Solid Edge part; units mm, degrees
sketch "Sketch1" plane through (0, 0, 0) normal (0, -1, 0) x (1, 0, 0)
  line L0 (2.75, 3) -> (2.75, 0)
  line L1 (2.75, 0) -> (1.8, 0)
  line L2 (1.8, 0) -> (1.5, -0.5196)
  line L3 (1.5, -0.5196) -> (1.5, -10)
  line L4 (1.5, -10) -> (0, -10)
  line L5 (1.25, 1.7) -> (0, 0.9783)
  line L6 (1.25, 3) -> (1.25, 1.7)
  line L7 (2.75, 3) -> (1.25, 3)
revolve "RevolvedProtrusion1" add sketch "Sketch1" angle 360 about axis through (0, 0, -6) along (0, 0, 1)
cosmetic_thread "Thread1"
chamfer "Chamfer_1" distance 0.25 angle 45 1 edges at (-1.5, 0, -10)
fillet "Round_1" radius 0.3 2 edges at (-2.75, 0, 0) (-2.75, 0, 3)
sketch "Sketch2" plane through (0, 0, 3) normal (0, 0, 1) x (0, 1, 0)
  line L0 (-1.25, 0.7217) -> (-1.25, -0.7217)
  line L1 (0, -1.4434) -> (-1.25, -0.7217)
  line L2 (1.25, -0.7217) -> (0, -1.4434)
  line L3 (1.25, 0.7217) -> (1.25, -0.7217)
  line L4 (0, 1.4434) -> (1.25, 0.7217)
  line L5 (-1.25, 0.7217) -> (0, 1.4434)
extrude "Cutout1" cut sketch "Sketch2" against normal up to vertex (1.3 mm away)
properties part number "STD-DIN912-M3x10" material "Galvanized steel"
Read the model definition and answer for the solid it produces. Units are mm, in the model's axes. A direction names the side the tool comes from. Round coordinates to 2 decimals unless told otherwise and drop trailing zeros. Write each loop counter-clockwise with the first axis right and the second up, starting at its lowest first coordinate (ties: lowest second). Pieces come first, ordered by that corner, then holes.
Q1. Find section A-A on z = -3.25. Determine the outline of the cut face in (x, y).
Values:
outline: circle Ø3 at (0, 0)
Q2. A tool of negligible diameter and unlimited length cuts with its end or side. For faces 1 (the face through (0, 0, -10)), 2 (the face through (1.08, 0.63, 2.36)), 3 (the face through (-1.5, -0.07, -5.2)), from which of +Z, -Z, +X, -X, +Y, -Y can it reach the whole face along a straight path? Write none if from no direction.
Values:
face 1: -Z, +X, -X, +Y, -Y
face 2: +Z
face 3: -Z
Q3. Straight lines are drawn through the part: line 1 (Z direction, x = 1.4, y = -1.9); line 2 (Z direction, x = 1.05, y = 0.95); line 3 (X direction, y = -0.1, z = -0.5). For each, find the intervals that lie inside material, in ascending order.
Values:
line 1: z = 0 to 3
line 2: z = -9.83 to 3
line 3: x = -1.51 to 1.51
Q4. Flat-ended cylindrical pins translate along their axes: P1, Ø1, axis at x = -1.5, z = -6, coming from the -Y side; P2, Ø1, axis at x = -1.5, y = -1.5, coming from the -Z side. Find the tip coordinate at first contact, or state that the pin passes through.
Values:
P1: stops at y = -1.12
P2: stops at z = -0.31
Q5. The mould has two halves that part along X. Classify faces 4 (the face through (0, -1.25, 2)), 5 (the face through (-0.596, 2.685, 1.483)), 6 (the face through (1.1, -1.1, 3)): released by +X, released by -X, zero draft, split by the parting line, or undercut.
Values:
face 4: undercut
face 5: split by the parting line
face 6: zero draft
